Solid Edge part; units mm, degrees
sketch "Sketch1" plane through (0, 0, 0) normal (0, 0, 1) x (1, 0, 0)
  circle A0 centre (0, 0) radius 1
  line L0 (-3, 25) -> (-3, 0)
  line L1 (3, 25) -> (3, 0)
  arc A1 (3, 25) -> (-3, 25) centre (0, 25) ccw
  arc A2 (-3, 0) -> (3, 0) centre (0, 0) ccw
  circle A3 centre (0, 25) radius 1
extrude "Protrusion1" add sketch "Sketch1" along normal blind 5
Could you check a few things on this model? Use its own coordinates, in mm. Round coordinates to 2 decimals unless told otherwise and drop trailing zeros. Write each loop counter-clockwise with the first axis right and the second up, starting at its lowest first coordinate (ties: lowest second). Pieces come first, ordered by that corner, then holes.
(1) Suppose I cut it at B-B on z = 2.5. Write out the boundary of the cut face in (x, y).
Findings below:
outline: (-3, 0) arc R3 ccw to (3, 0) - (3, 25) arc R3 ccw to (-3, 25) - close; hole circle Ø2 at (0, 0); hole circle Ø2 at (0, 25)
(2) Suppose I cut it at C-C on x = 1.75. Write out the boundary of the cut face in (y, z).
Findings below:
outline: (-2.44, 0) - (27.44, 0) - (27.44, 5) - (-2.44, 5) - close
(3) Suppose I cut it at A-A on x = 0. Write out the boundary of the cut face in (y, z).
Findings below:
outline: (-3, 0) - (-1, 0) - (-1, 5) - (-3, 5) - close; (1, 0) - (24, 0) - (24, 5) - (1, 5) - close; (26, 0) - (28, 0) - (28, 5) - (26, 5) - close
(4) Thinking about a two-plate mould opening in X: for faces 1 (the face through (0, -3, 2)), 2 (the face through (0, 26, 2)), 3 (the face through (3, 13, 2)), 4 (the face through (-3, 13, 2)), which applies, +X half, -X half, draft (parallel to the pull), parting line (faces both ways), or undercut?
Findings below:
face 1: parting line
face 2: undercut
face 3: +X half
face 4: -X half
(5) If I drill on probe 1 along Y at (x, z) = (0, 1.45); probe 2 along Y at (x, z) = (0.75, 3.7); probe 3 along Y at (x, z) = (-2.5, 3.35), over which ranges is the centre line in solid material (lowest first)?
Findings below:
probe 1: y = -3 to -1, 1 to 24, 26 to 28
probe 2: y = -2.9 to -0.66, 0.66 to 24.34, 25.66 to 27.9
probe 3: y = -1.66 to 26.66
